Source: CAD feature listing. Evaluate the final solid. Frame: model axes, mm. A direction names the side the tool comes from. Give positions to 0.01 mm unless a question says otherwise; leave off trailing zeros. Write each loop counter-clockwise with the first axis right and the second up, starting at its lowest first coordinate (ties: lowest second). Pieces come first, ordered by that corner, then holes. Notation, with made-up numbers: M 17,52 L 35,52 A14 ccw 35,66 Z; hole C 9,3 d6. An arc over 180 degrees is marked long. Use CSV: the item, a comma, the result in double quotes. Start each with the question number.
from build123d import *

# Parameters (mm, degrees)
F1_DEPTH        = 6.4
F1_COPIES_COUNT = 3


# Not quite as in the source:
# - a feature of the source that left no trace in its solid (it failed there, or was rolled back) is left out
# - a pattern or mirror of a feature is missing from the dataset's text; its kind, count and spacing are read off the source's solid


with BuildPart() as f1:
    # F0 (on Front) → F1 (new body)
    with BuildSketch(Plane.XZ):
        with BuildLine():
            Line((10.9347, -15), (14, -15))
            ThreePointArc((14, -15), (0, -1), (-14, -15))
            Line((-14, -15), (-10.9347, -15))
            ThreePointArc((-10.9347, -15), (0, -4.0653), (10.9347, -15))
        make_face()
        with BuildLine():
            ThreePointArc((-14, -15), (0, -29), (14, -15))
            Line((14, -15), (10.9347, -15))
            ThreePointArc((10.9347, -15), (0, -25.9347), (-10.9347, -15))
            Line((-10.9347, -15), (-14, -15))
        make_face()
        with BuildLine():
            ThreePointArc((-14, -15), (0, -1), (14, -15))
            Line((14, -15), (14, 15))
            ThreePointArc((14, 15), (0, 1), (-14, 15))
            Line((-14, 15), (-14, -15))
        make_face()
        with BuildLine():
            ThreePointArc((-14, 15), (0, 1), (14, 15))
            Line((14, 15), (10.9347, 15))
            ThreePointArc((10.9347, 15), (0, 4.0653), (-10.9347, 15))
            Line((-10.9347, 15), (-14, 15))
        make_face()
        with BuildLine():
            Line((10.9347, 15), (14, 15))
            ThreePointArc((14, 15), (0, 29), (-14, 15))
            Line((-14, 15), (-10.9347, 15))
            ThreePointArc((-10.9347, 15), (0, 25.9347), (10.9347, 15))
        make_face()
    extrude(amount=F1_DEPTH)

    # F1_copies: F1 ×3 about axis
    f1_copies_axis = Axis((0, 0, 15), (0, 1, 0))


with BuildPart() as f1_1:
    add(f1.part)
    for i in range(1, F1_COPIES_COUNT):
        add(f1.part.rotate(f1_copies_axis, i * 360 / F1_COPIES_COUNT))


solid = f1_1.part
Item 1: Section B-B (x = -3). Return the cut outline in (y, z), plus the area to 3 significant figures.
Item 2: Contact query for flat-ended pins moving along their axis: pin 1 Ø1.5 at (x, y) = (16.5, -5) entering from -Z; pin 2 Ø1.9 at (y, z) = (-4, -8.5) entering from +X. Output: stop coordinate, or through.
Item 3: Pull-direction query (X, two-part tool) for faces 1 (the flat face through (12, -6.4, 15)), 2 (the flat face through (-23.62, -3.16, 12.47)), 3 (the cylindrical face through (-36.905, -3.155, 29.519)); classes: released by +X, released by -X, zero draft, split by the parting line, or undercut.
Item 4: Section D-D (x = 28). Return the cut outline in (y, z).
Item 5: Section C-C (z = 15). Return the cut outline in (x, y), plus the area to 3 significant figures.
Item 6: Material intervals for probe 1 along X at (y, z) = (-1.5, 28.5); probe 2 along Z at (x, y) = (-2, -5.5); probe 3 along X at (y, z) = (-3.25, 26.5), sorted ascending.
Item 7: Set-up query: faces 4 (the flat face through (9.62, -3.16, 36.72)), 5 (the cylindrical face through (0, -3, -29)), 6 (the flat face through (-14, -3, -4)), 7 (the flat face through (14, -3, -4)). Return all of +Z, -Z, +X, -X, +Y, -Y with unobstructed straight access to the full face (end or side cutting, diameter ignored); none if empty.
Item 8: Section A-A (z = 30). Return the cut outline in (x, y), plus the area to 3 significant figures.
Output values:
1,outline,"M -6.4,-28.67 L 0,-28.67 L 0,-25.52 L -6.4,-25.52 Z; M -6.4,-4.48 L 0,-4.48 L 0,4.48 L -6.4,4.48 Z; M -6.4,25.52 L 0,25.52 L 0,32.9 L -6.4,32.9 Z"
1,area,"125 mm2"
2,pin 1,"stops at z = 7.93"
2,pin 2,"stops at x = 14"
3,face 1,"zero draft"
3,face 2,"released by -X"
3,face 3,"undercut"
4,outline,"M -6.4,15 L 0,15 L 0,19.25 L -6.4,19.25 Z; M -6.4,40.75 L 0,40.75 L 0,43.85 L -6.4,43.85 Z"
5,outline,"M -28,-6.4 L -10.93,-6.4 L -10.93,0 L -28,0 Z; M 10.93,-6.4 L 28,-6.4 L 28,0 L 10.93,0 Z"
5,area,"218 mm2"
6,probe 1,"x = -39.9 to -36.81, -15.15 to 15.15, 36.81 to 39.9"
6,probe 2,"z = -28.86 to -25.75, -4.25 to 4.25, 25.75 to 32.32"
6,probe 3,"x = -39.54 to -36.34, -15.62 to 15.62, 36.34 to 39.54"
7,face 4,"+Z, +Y, -Y"
7,face 5,"-Z, +Y, -Y"
7,face 6,"-Z, -X, +Y, -Y"
7,face 7,"-Z, +X, +Y, -Y"
8,outline,"M -39.98,-6.4 L -36.92,-6.4 L -36.92,0 L -39.98,0 Z; M -15.05,-6.4 L 15.05,-6.4 L 15.05,0 L -15.05,0 Z; M 36.92,-6.4 L 39.98,-6.4 L 39.98,0 L 36.92,0 Z"
8,area,"232 mm2"
